CAD build for the part. Positions are in the model's coordinates, mm. Face numbers are marked on the shaded views. A direction names the side the tool comes from. Give positions to 0.01 mm unless a question says otherwise; leave off trailing zeros. Loops run counter-clockwise (first coordinate to the right, second up) from the corner with the lowest first, then second, coordinate; pieces in that order, holes last.
Item 1: Saw through at D-D on x = 23. Give the cut face in (y, z), plus the area to 3 significant figures.
Item 2: Which spindle directions (+Z, -Z, +X, -X, +Y, -Y) get a long thin tool onto all of the face, cutting with end or side? Do the marked faces 4, 5 and 6. Say none if no direction does.
Item 3: Saw through at C-C on y = 11.75. Give the cut face in (x, z).
Item 4: Saw through at B-B on y = 3. Give the cut face in (x, z).
Item 5: Probe probe 1 along Z at (x, y) = (26.3, 0.35); probe 2 along Y at (x, z) = (-24, 23.5); probe 3 along Z at (x, y) = (-15, 3.5). List the from-to ranges inside material, lowest first.
Item 6: Saw through at A-A on z = 50.4. Give the cut face in (x, y), plus the area to 3 significant figures.
Item 7: Drop flat-ended pins along their axis: P1, Ø4, axis at x = -24, y = 7.5, coming from the +Z side; P2, Ø6, axis at x = -4.5, y = 8, coming from the -Z side; P3, Ø9.5, axis at x = -8.5, z = -42.5, coming from the +Y side. Give the stop position or say it passes through.
Item 8: Mould opens along X. For the marked faces 1, 2 and 3 say: released by +X, released by -X, zero draft, split by the parting line, or undercut.
Autodesk Inventor part; units mm, degrees
ref_plane "YZ Plane" through (0, 0, 0) normal (1, 0, 0) x (0, 1, 0)
ref_plane "XZ Plane" through (0, 0, 0) normal (0, 1, 0) x (-1, 0, 0)
ref_plane "XY Plane" through (0, 0, 0) normal (0, 0, 1) x (1, 0, 0)
sketch "Sketch1" plane through (0, 0, 0) normal (0, 1, 0) x (-1, 0, 0)
  line L0 (-30, 54.1) -> (30, 54.1)
  line L1 (30, 54.1) -> (30, -54.1)
  line L2 (30, -54.1) -> (-30, -54.1)
  line L3 (-30, -54.1) -> (-30, 54.1)
  line L4 (-30, 54.1) -> (30, -54.1) construction
  line L5 (30, 54.1) -> (-30, -54.1) construction
  circle A0 centre (26.3, 50.4) radius 1.5
  line L6 (0, 0) -> (11.9593, 0)
  line L7 (0, 0) -> (0, 9.8578)
  circle A1 centre (26.3, -50.4) radius 1.5
  circle A2 centre (-26.3, 50.4) radius 1.5
  circle A3 centre (-26.3, -50.4) radius 1.5
  dimension "d0" = 60
  dimension "d1" = 108.2
  dimension "d2" = 3.7
  dimension "d3" = 3.7
  dimension "d4" = 3
extrude "Extrusion1" add sketch "Sketch1" along normal blind 1.5
sketch "Sketch2" plane through (0, 1.5, 0) normal (0, 1, 0) x (1, 0, 0)
  line L0 (30, 54.1) -> (-30, 54.1)
  line L1 (-30, 54.1) -> (-30, -54.1)
  line L2 (-30, -54.1) -> (30, -54.1)
  line L3 (30, -54.1) -> (30, 54.1)
  circle A0 centre (26.3, 50.4) radius 1.5
  circle A1 centre (26.3, -50.4) radius 1.5
  circle A2 centre (-26.3, 50.4) radius 1.5
  circle A3 centre (-26.3, -50.4) radius 1.5
  line L4 (7.6, -45.3) -> (-7.6, -45.3)
  line L5 (-7.6, -45.3) -> (-7.6, -43.1)
  line L6 (-7.6, -43.1) -> (7.6, -43.1)
  line L7 (7.6, -43.1) -> (7.6, -45.3)
  line L8 (7.6, -45.3) -> (-7.6, -43.1) construction
  line L9 (-7.6, -45.3) -> (7.6, -43.1) construction
  point P0 (0, 0)
  point P1 (0, -44.2)
  point P2 (0, -54.1)
  dimension "d7" = 2.2
  dimension "d8" = 15.2
  dimension "d9" = 11
extrude "Extrusion2" add sketch "Sketch2" along normal blind 8 contours L4 L5 L6 L7
sketch "Sketch3" plane through (0, 0, 0) normal (0, -1, 0) x (1, 0, 0)
  circle A0 centre (16.0331, -17.0211) radius 2.267
  circle A1 centre (-4.9851, -17.0211) radius 1.9033
  circle A2 centre (-1.7515, 17.0211) radius 2.2093
  circle A3 centre (16.0331, 36.153) radius 3.7001
  point P0 (0, 0)
extrude "Extrusion3" add sketch "Sketch3" along normal blind 2
sketch "Sketch4" plane through (0, 1.5, 0) normal (0, 1, 0) x (1, 0, 0)
  circle A0 centre (-6, 24.6) radius 5
  circle A1 centre (6, 24.6) radius 5
  line L0 (30, 54.1) -> (-30, 54.1)
  line L1 (-6, 24.6) -> (6, 24.6)
  point P0 (0, 0)
  point P1 (0, 24.6)
  point P2 (0, 54.1)
  dimension "d14" = 10
  dimension "d15" = 29.5
  dimension "d16" = 12
extrude "Extrusion4" add sketch "Sketch4" along normal blind 22
sketch "Sketch5" plane through (0, 1.5, 0) normal (0, 1, 0) x (1, 0, 0)
  circle A0 centre (6, 24.6) radius 5
  circle A1 centre (-6, 24.6) radius 5
  line L0 (7.6, -43.1) -> (7.6, -45.3)
  line L1 (7.6, -45.3) -> (-7.6, -45.3)
  line L2 (-7.6, -45.3) -> (-7.6, -43.1)
  line L3 (-7.6, -43.1) -> (7.6, -43.1)
  line L4 (30, 54.1) -> (-30, 54.1)
  line L5 (-30, 54.1) -> (-30, -54.1)
  line L6 (-30, -54.1) -> (30, -54.1)
  line L7 (30, -54.1) -> (30, 54.1)
  circle A2 centre (26.3, 50.4) radius 1.5
  circle A3 centre (26.3, -50.4) radius 1.5
  circle A4 centre (-26.3, 50.4) radius 1.5
  circle A5 centre (-26.3, -50.4) radius 1.5
  line L8 (26, 33.6) -> (-26, 33.6)
  line L9 (-26, 33.6) -> (-26, 45.6)
  line L10 (-26, 45.6) -> (26, 45.6)
  line L11 (26, 45.6) -> (26, 33.6)
  line L12 (26, 33.6) -> (-26, 45.6) construction
  line L13 (-26, 33.6) -> (26, 45.6) construction
  point P0 (0, 0)
  point P1 (0, 39.6)
  dimension "d19" = 52
  dimension "d20" = 12
  dimension "d21" = 8.5
extrude "Extrusion5" add sketch "Sketch5" along normal blind 12.5 contours L8 L9 L10 L11
properties part number "DRIVER" material "Steel, Mild, Welded"
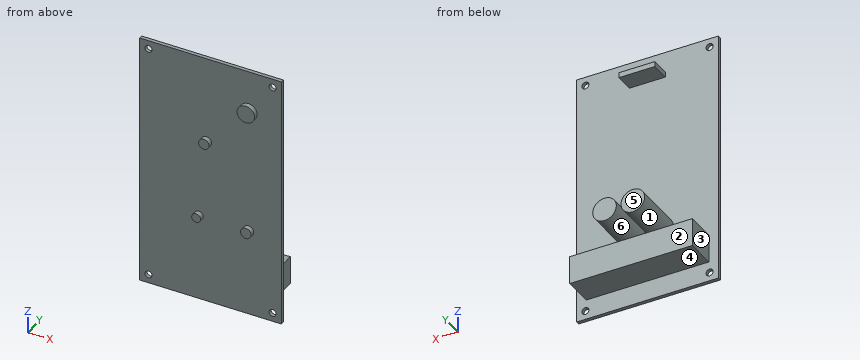
Results below:
1. outline: (0, -54.1) - (1.5, -54.1) - (1.5, -45.6) - (14, -45.6) - (14, -33.6) - (1.5, -33.6) - (1.5, 54.1) - (0, 54.1) - close
1. area: 312 mm2
2. face 4: -Z, +X, -X, +Y
2. face 5: +Z, -Z, +X, -X, +Y
2. face 6: +Y
3. outline: (-26, -45.6) - (26, -45.6) - (26, -33.6) - (-26, -33.6) - close; circle Ø10 at (-6, -24.6); circle Ø10 at (6, -24.6)
4. outline: (-26, -45.6) - (26, -45.6) - (26, -33.6) - (-26, -33.6) - close; circle Ø10 at (-6, -24.6); (-7.6, 43.1) - (7.6, 43.1) - (7.6, 45.3) - (-7.6, 45.3) - close; circle Ø10 at (6, -24.6)
5. probe 1: z = -54.1 to -51.9, -48.9 to 48.9, 51.9 to 54.1
5. probe 2: y = 0 to 1.5
5. probe 3: z = -45.6 to -33.6
6. outline: (-30, 0) - (-27.8, 0) - (-27.8, 1.5) - (-30, 1.5) - close; (-24.8, 0) - (24.8, 0) - (24.8, 1.5) - (-24.8, 1.5) - close; (27.8, 0) - (30, 0) - (30, 1.5) - (27.8, 1.5) - close
6. area: 81.0 mm2
7. P1: stops at z = -33.6
7. P2: stops at z = -45.6
7. P3: stops at y = 14
8. face 1: undercut
8. face 2: zero draft
8. face 3: released by -X
